For this review, take the finished solid that the model builds, in its own axes (mm). A direction names the side the tool comes from. Give positions to 0.01 mm unless a question says otherwise; leave off trailing zeros. Order: outer loops, then holes, each group sorted by start corner. A loop starts at its lowest first (then second) coordinate and runs counter-clockwise, first axis right, second up.
Item 1: For P1, Ø17, axis at x = -41.275, z = -206.375, coming from the -Y side; P2, Ø6.5, axis at x = -85.5, z = -194, coming from the -Y side; P3, Ø5, axis at x = -71.44, z = 217.49, coming from the -Y side, all flat-tipped, find the tip position at first contact; note any pin that passes through.
Item 2: Consider section B-B (x = -49). Give the boundary of the cut face in (y, z), plus the area to 3 significant figures.
Item 3: Machinability: for faces 1 (the cylindrical face through (-28.08, -15.23, 211.85)), 2 (the flat face through (54, -4.762, -214)), 3 (the flat face through (-84.2, -17.462, 187.7)), which of the approach directions +Z, -Z, +X, -X, +Y, -Y give a long, thin tool a straight path to every point of the face, cutting with its end or side? Answer none if there is none.
Item 4: The part is to be moulded in two halves that separate along X. For faces 4 (the flat face through (-1, -13, -228.6)), 5 (the cylindrical face through (-89.49, -21.49, 187.98)), say which applies: released by +X, released by -X, zero draft, split by the parting line, or undercut.
Item 5: For probe 1 along X at (y, z) = (-16, -101.6); probe 2 along X at (y, z) = (-10, -208); probe 3 along Z at (x, y) = (40, -7.75), list the stretches that pass through material, from the lowest coordinate up.
Item 6: Consider section A-A (x = 0). Give the boundary of the cut face in (y, z).
```python
from build123d import *

# Parameters (mm, degrees)
SKETCH1_W            = 187.325
SKETCH1_H            = 25.4
BASE_EXTRUDE_DEPTH   = 228.6
CBORE1_D             = 8.4328
CBORE1_CBORE_D       = 13.49375
CBORE1_CBORE_DEPTH   = 7.9375
CBORE2_D             = 8.4328
CBORE2_CBORE_D       = 13.49375
CBORE2_CBORE_DEPTH   = 7.9375
CBORE3_D             = 8.4328
CBORE3_CBORE_D       = 13.49375
CBORE3_CBORE_DEPTH   = 7.9375
CBORE4_D             = 8.4328
CBORE4_CBORE_D       = 13.49375
CBORE4_CBORE_DEPTH   = 7.9375
CUT_EXTRUDE1_DEPTH   = 3.175
MIRROR2_COPY_1_DEPTH = 3.175
GUIDE1_START         = -25.4
GUIDE1_OUTLINE_R     = 14.2875
GUIDE1_DEPTH         = 25.4
CBORE5_START         = -25.4
CBORE5_OUTLINE_R     = 14.2875
CBORE5_OUTLINE_R_2   = 4.2164
CBORE5_DEPTH         = 25.4
CBORE5_START_2       = -4.7625
CBORE5_2_OUTLINE_R   = 16.66875
CBORE5_2_OUTLINE_R_2 = 14.2875
CBORE5_2_DEPTH       = 4.7625
CBORE5_3_OUTLINE_R   = 6.746875
CBORE5_3_OUTLINE_R_2 = 4.2164
CBORE5_3_DEPTH       = 7.9375
CBORE6_D             = 8.4328
CBORE6_CBORE_D       = 13.49375
CBORE6_CBORE_DEPTH   = 7.9375


# Read off the part's stored shape, not the designer's step: Guide1, CBORE5
with BuildPart() as part:
    # Sketch1 → Base-Extrude (new, symmetric)
    with BuildSketch(Plane.XY):
        with Locations((0, -12.7)):
            Rectangle(SKETCH1_W, SKETCH1_H)
    extrude(amount=BASE_EXTRUDE_DEPTH, both=True)

    # CBORE1 (through all)
    with Locations(Plane.XZ.offset(25.4)):
        with Locations((84.1375, -192.0875)):
            CounterBoreHole(CBORE1_D / 2, CBORE1_CBORE_D / 2, CBORE1_CBORE_DEPTH)

    # CBORE2 (through all)
    with Locations(Plane.XZ.offset(25.4)):
        with Locations((84.1375, 192.0875)):
            CounterBoreHole(CBORE2_D / 2, CBORE2_CBORE_D / 2, CBORE2_CBORE_DEPTH)

    # CBORE3 (through all)
    with Locations(Plane.XZ.offset(25.4)):
        with Locations((-84.1375, 192.0875)):
            CounterBoreHole(CBORE3_D / 2, CBORE3_CBORE_D / 2, CBORE3_CBORE_DEPTH)

    # CBORE4 (through all)
    with Locations(Plane.XZ.offset(25.4)):
        with Locations((-84.1375, -192.0875)):
            CounterBoreHole(CBORE4_D / 2, CBORE4_CBORE_D / 2, CBORE4_CBORE_DEPTH)

    # Sketch3 → Cut-Extrude1 (cut)
    with BuildSketch(Plane(origin=(0, 0, 0), x_dir=(-1, 0, 0), z_dir=(0, 1, 0))):
        Polygon((-86.927307909, 228.6), (-93.6625, 221.864807909), (-93.6625, 228.6), align=None)
    cut_extrude1 = extrude(amount=-CUT_EXTRUDE1_DEPTH, mode=Mode.SUBTRACT)

    # Mirror1: Cut-Extrude1 across plane
    add(cut_extrude1.mirror(Plane(origin=(0, 0, 0), x_dir=(0, 0, 1), z_dir=(1, 0, 0))), mode=Mode.SUBTRACT)

    # Mirror2: Cut-Extrude1 across plane
    add(cut_extrude1.mirror(Plane.XY), mode=Mode.SUBTRACT)

    # Mirror2 copy 1 sketch → Mirror2 copy 1 (cut)
    with BuildSketch(Plane(origin=(0, 0, 0), x_dir=(1, 0, 0), z_dir=(0, 1, 0))):
        Polygon((-86.927307909, 228.6), (-93.6625, 221.864807909), (-93.6625, 228.6), align=None)
    extrude(amount=-MIRROR2_COPY_1_DEPTH, mode=Mode.SUBTRACT)

    # SP1rev → SP1 (revolve, cut)
    with BuildSketch(Plane(origin=(-71.4375, -25.4, -217.4875), x_dir=(0, 0, -1), z_dir=(1, 0, 0))):
        Polygon((0, 0), (0, 18.259649766), (3.968746562, 15.87498625), (3.968746562, 0.002539998), (3.968746563, 0), align=None)
    revolve(axis=Axis((-71.4375, -31.75, -217.4875), (0, 1, 0)), mode=Mode.SUBTRACT)

    # SP2rev → SP2 (revolve, cut)
    with BuildSketch(Plane(origin=(-71.4375, -25.4, 217.4875), x_dir=(0, 0, -1), z_dir=(1, 0, 0))):
        Polygon((0, 0), (0, 18.259649766), (3.968746562, 15.87498625), (3.968746562, 0.002539998), (3.968746563, 0), align=None)
    sp2 = revolve(axis=Axis((-71.4375, -31.75, 217.4875), (0, 1, 0)), mode=Mode.SUBTRACT)

    # SP3rev → SP3 (revolve, cut)
    with BuildSketch(Plane(origin=(-71.4375, -25.4, 0.218909537), x_dir=(0, 0, -1), z_dir=(1, 0, 0))):
        Polygon((0, 0), (0, 18.259649766), (3.968746562, 15.87498625), (3.968746562, 0.002539998), (3.968746563, 0), align=None)
    sp3 = revolve(axis=Axis((-71.4375, -31.75, 0.218909537), (0, 1, 0)), mode=Mode.SUBTRACT)

    # SP4rev → SP4 (revolve, cut)
    with BuildSketch(Plane(origin=(-71.4375, -25.4, 101.6), x_dir=(0, 0, -1), z_dir=(1, 0, 0))):
        Polygon((0, 0), (0, 18.259649766), (3.968746562, 15.87498625), (3.968746562, 0.002539998), (3.968746563, 0), align=None)
    sp4 = revolve(axis=Axis((-71.4375, -31.75, 101.6), (0, 1, 0)), mode=Mode.SUBTRACT)

    # SP5rev → SP5 (revolve, cut)
    with BuildSketch(Plane(origin=(-71.4375, -25.4, -101.6), x_dir=(0, 0, -1), z_dir=(1, 0, 0))):
        Polygon((0, 0), (0, 18.259649766), (3.968746562, 15.87498625), (3.968746562, 0.002539998), (3.968746563, 0), align=None)
    sp5 = revolve(axis=Axis((-71.4375, -31.75, -101.6), (0, 1, 0)), mode=Mode.SUBTRACT)

    # SP6rev → SP6 (revolve, cut)
    with BuildSketch(Plane(origin=(71.4375, -25.4, -214.3125), x_dir=(0, 0, -1), z_dir=(1, 0, 0))):
        Polygon((0, 0), (0, 18.259649766), (3.968746562, 15.87498625), (3.968746562, 0.002539998), (3.968746563, 0), align=None)
    revolve(axis=Axis((71.4375, -31.75, -214.3125), (0, 1, 0)), mode=Mode.SUBTRACT)

    # Guide1 outline → Guide1 (cut)
    with BuildSketch(Plane(origin=(0, 0, 0), x_dir=(1, 0, 0), z_dir=(0, 1, 0)).offset(GUIDE1_START)):
        with Locations((41.275, 206.375)):
            Circle(GUIDE1_OUTLINE_R)
    extrude(amount=GUIDE1_DEPTH, mode=Mode.SUBTRACT)

    # CBORE5 outline → CBORE5 (cut)
    with BuildSketch(Plane(origin=(0, 0, 0), x_dir=(1, 0, 0), z_dir=(0, 1, 0)).offset(CBORE5_START)):
        with Locations((0, -206.375)):
            Circle(CBORE5_OUTLINE_R)
        with Locations((0, 206.375)):
            Circle(CBORE5_OUTLINE_R)
        with Locations((-41.275, 206.375)):
            Circle(CBORE5_OUTLINE_R)
        with Locations((-41.275, -206.375)):
            Circle(CBORE5_OUTLINE_R)
        with Locations((41.275, -206.375)):
            Circle(CBORE5_OUTLINE_R)
        with Locations((84.1375, 0)):
            Circle(CBORE5_OUTLINE_R_2)
    extrude(amount=CBORE5_DEPTH, mode=Mode.SUBTRACT)

    # CBORE5 2 outline → CBORE5 2 (cut)
    # profile 1 of 6: a face of its own
    with BuildSketch(Plane(origin=(0, 0, 0), x_dir=(1, 0, 0), z_dir=(0, 1, 0)).offset(CBORE5_START_2)):
        with Locations((41.275, 206.375)):
            Circle(CBORE5_2_OUTLINE_R)
        with Locations((41.275, 206.375)):
            Circle(CBORE5_2_OUTLINE_R_2, mode=Mode.SUBTRACT)
    # profile 2 of 6: a face of its own
    with BuildSketch(Plane(origin=(0, 0, 0), x_dir=(1, 0, 0), z_dir=(0, 1, 0)).offset(CBORE5_START_2)):
        with Locations((41.275, -206.375)):
            Circle(CBORE5_2_OUTLINE_R)
        with Locations((41.275, -206.375)):
            Circle(CBORE5_2_OUTLINE_R_2, mode=Mode.SUBTRACT)
    # profile 3 of 6: a face of its own
    with BuildSketch(Plane(origin=(0, 0, 0), x_dir=(1, 0, 0), z_dir=(0, 1, 0)).offset(CBORE5_START_2)):
        with Locations((-41.275, -206.375)):
            Circle(CBORE5_2_OUTLINE_R)
        with Locations((-41.275, -206.375)):
            Circle(CBORE5_2_OUTLINE_R_2, mode=Mode.SUBTRACT)
    # profile 4 of 6: a face of its own
    with BuildSketch(Plane(origin=(0, 0, 0), x_dir=(1, 0, 0), z_dir=(0, 1, 0)).offset(CBORE5_START_2)):
        with Locations((-41.275, 206.375)):
            Circle(CBORE5_2_OUTLINE_R)
        with Locations((-41.275, 206.375)):
            Circle(CBORE5_2_OUTLINE_R_2, mode=Mode.SUBTRACT)
    # profile 5 of 6: a face of its own
    with BuildSketch(Plane(origin=(0, 0, 0), x_dir=(1, 0, 0), z_dir=(0, 1, 0)).offset(CBORE5_START_2)):
        with Locations((0, 206.375)):
            Circle(CBORE5_2_OUTLINE_R)
        with Locations((0, 206.375)):
            Circle(CBORE5_2_OUTLINE_R_2, mode=Mode.SUBTRACT)
    # profile 6 of 6: a face of its own
    with BuildSketch(Plane(origin=(0, 0, 0), x_dir=(1, 0, 0), z_dir=(0, 1, 0)).offset(CBORE5_START_2)):
        with Locations((0, -206.375)):
            Circle(CBORE5_2_OUTLINE_R)
        with Locations((0, -206.375)):
            Circle(CBORE5_2_OUTLINE_R_2, mode=Mode.SUBTRACT)
    extrude(amount=CBORE5_2_DEPTH, mode=Mode.SUBTRACT)

    # CBORE5 3 outline → CBORE5 3 (cut)
    with BuildSketch(Plane(origin=(0, 0, 0), x_dir=(1, 0, 0), z_dir=(0, 1, 0)).offset(CBORE5_START)):
        with Locations((84.1375, 0)):
            Circle(CBORE5_3_OUTLINE_R)
        with Locations((84.1375, 0)):
            Circle(CBORE5_3_OUTLINE_R_2, mode=Mode.SUBTRACT)
    extrude(amount=CBORE5_3_DEPTH, mode=Mode.SUBTRACT)

    # CBORE6 (through all)
    with Locations(Plane(origin=(-174.013483356, -25.4, 84.713166839), x_dir=(1, 0, 0), z_dir=(0, -1, 0))):
        with Locations((89.875983356, -84.713166839)):
            CounterBoreHole(CBORE6_D / 2, CBORE6_CBORE_D / 2, CBORE6_CBORE_DEPTH)

    # Mirror3: SP3 across plane
    add(sp3.mirror(Plane(origin=(0, 0, 0), x_dir=(0, 0, 1), z_dir=(1, 0, 0))), mode=Mode.SUBTRACT)

    # Mirror4: SP4, SP5 across plane
    add(sp4.mirror(Plane(origin=(0, 0, 0), x_dir=(0, 0, 1), z_dir=(1, 0, 0))), mode=Mode.SUBTRACT)
    add(sp5.mirror(Plane(origin=(0, 0, 0), x_dir=(0, 0, 1), z_dir=(1, 0, 0))), mode=Mode.SUBTRACT)

    # Mirror5: SP2 across plane
    add(sp2.mirror(Plane(origin=(0, 0, 0), x_dir=(0, 0, 1), z_dir=(1, 0, 0))), mode=Mode.SUBTRACT)


solid = part.part
```
Resolved:
1. P1: passes through
1. P2: stops at y = -17.46
1. P3: stops at y = -8.64
2. outline: (-25.4, -228.6) - (0, -228.6) - (0, -221.15) - (-4.76, -221.15) - (-4.76, -218.39) - (-25.4, -218.39) - close; (-25.4, -194.36) - (-4.76, -194.36) - (-4.76, -191.6) - (0, -191.6) - (0, 191.6) - (-4.76, 191.6) - (-4.76, 194.36) - (-25.4, 194.36) - close; (-25.4, 218.39) - (-4.76, 218.39) - (-4.76, 221.15) - (0, 221.15) - (0, 228.6) - (-25.4, 228.6) - close
2. area: 10,300 mm2
3. face 1: +Y, -Y
3. face 2: +Y
3. face 3: -Y
4. face 4: zero draft
4. face 5: undercut
5. probe 1: x = -93.66 to -75.41, -67.47 to 67.47, 75.41 to 93.66
5. probe 2: x = -93.66 to -55.47, -27.08 to -14.19, 14.19 to 27.08, 55.47 to 93.66
5. probe 3: z = -228.6 to -220.61, -192.14 to 192.14, 220.61 to 228.6
6. outline: (-25.4, -228.6) - (0, -228.6) - (0, -223.04) - (-4.76, -223.04) - (-4.76, -220.66) - (-25.4, -220.66) - close; (-25.4, -192.09) - (-4.76, -192.09) - (-4.76, -189.71) - (0, -189.71) - (0, 189.71) - (-4.76, 189.71) - (-4.76, 192.09) - (-25.4, 192.09) - close; (-25.4, 220.66) - (-4.76, 220.66) - (-4.76, 223.04) - (0, 223.04) - (0, 228.6) - (-25.4, 228.6) - close
